```python
from build123d import *

# Parameters (mm, degrees)
SKETCH_1_W          = 35
SKETCH_1_H          = 100
EXTRUDE_1_DEPTH     = 100
SKETCH_1_3_W        = 35
SKETCH_1_3_H        = 100
EXTRUDE_2_DEPTH     = 120
SKETCH_1_4_W        = 35
SKETCH_1_4_H        = 100
EXTRUDE_3_DEPTH     = 140
SKETCH_1_5_W        = 195.279005499
SKETCH_1_5_H        = 100
EXTRUDE_4_DEPTH     = 160
SKETCH_1_6_W        = 60
SKETCH_1_6_H        = 100
EXTRUDE_5_DEPTH     = 160
SKETCH_17_R         = 3.5
CUT_EXTRUDE_4_DEPTH = 25
SKETCH_18_R         = 3.5
CUT_EXTRUDE_5_DEPTH = 25


with BuildPart() as part:
    # Sketch 1 → Extrude 1 (new body)
    with BuildSketch(Plane(origin=(0, 0, 0), x_dir=(1, 0, 0), z_dir=(0, 1, 0))):
        with Locations((17.5, 50)):
            Rectangle(SKETCH_1_W, SKETCH_1_H)
    extrude(amount=EXTRUDE_1_DEPTH)

    # Sketch 1_3 → Extrude 2 (add)
    with BuildSketch(Plane(origin=(0, 0, 0), x_dir=(1, 0, 0), z_dir=(0, 1, 0))):
        with Locations((52.5, 50)):
            Rectangle(SKETCH_1_3_W, SKETCH_1_3_H)
    extrude(amount=EXTRUDE_2_DEPTH)

    # Sketch 1_4 → Extrude 3 (add)
    with BuildSketch(Plane(origin=(0, 0, 0), x_dir=(1, 0, 0), z_dir=(0, 1, 0))):
        with Locations((87.5, 50)):
            Rectangle(SKETCH_1_4_W, SKETCH_1_4_H)
    extrude(amount=EXTRUDE_3_DEPTH)

    # Sketch 1_5 → Extrude 4 (add)
    with BuildSketch(Plane(origin=(0, 0, 0), x_dir=(1, 0, 0), z_dir=(0, 1, 0))):
        with Locations((202.639502749, 50)):
            Rectangle(SKETCH_1_5_W, SKETCH_1_5_H)
    extrude(amount=EXTRUDE_4_DEPTH)

    # Sketch 1_6 → Extrude 5 (add)
    with BuildSketch(Plane(origin=(0, 0, 0), x_dir=(1, 0, 0), z_dir=(0, 1, 0))):
        with Locations((330.279005499, 50)):
            Rectangle(SKETCH_1_6_W, SKETCH_1_6_H)
    extrude(amount=EXTRUDE_5_DEPTH)

    # Sketch 17 → Cut-Extrude 4 (cut)
    with BuildSketch(Plane(origin=(0, 120, 0), x_dir=(1, 0, 0), z_dir=(0, 1, 0))):
        with Locations(Location((53.859111314, 83.458390634, 0), (0, 0, 270))):
            Circle(SKETCH_17_R)
        with Locations(Location((53.859111314, 62.301745528, 0), (0, 0, 270))):
            Circle(SKETCH_17_R)
        with Locations(Location((53.859111314, 41.942908687, 0), (0, 0, 270))):
            Circle(SKETCH_17_R)
        with Locations(Location((53.859111314, 19.312140714, 0), (0, 0, 270))):
            Circle(SKETCH_17_R)
    extrude(amount=-CUT_EXTRUDE_4_DEPTH, mode=Mode.SUBTRACT)

    # Sketch 18 → Cut-Extrude 5 (cut)
    with BuildSketch(Plane(origin=(0, 140, 0), x_dir=(1, 0, 0), z_dir=(0, 1, 0))):
        with Locations(Location((87.572175359, 84.853566518, 0), (0, 0, 270))):
            Circle(SKETCH_18_R)
        with Locations(Location((87.572175359, 63.696921411, 0), (0, 0, 270))):
            Circle(SKETCH_18_R)
        with Locations(Location((87.572175359, 43.338084571, 0), (0, 0, 270))):
            Circle(SKETCH_18_R)
        with Locations(Location((87.572175359, 20.707316598, 0), (0, 0, 270))):
            Circle(SKETCH_18_R)
    extrude(amount=-CUT_EXTRUDE_5_DEPTH, mode=Mode.SUBTRACT)


solid = part.part
```
Design review of the part built by this model. Coordinates are the model's own, in mm. A direction names the side the tool comes from. Round coordinates to 2 decimals unless told otherwise and drop trailing zeros. Order: outer loops, then holes, each group sorted by start corner. A loop starts at its lowest first (then second) coordinate and runs counter-clockwise, first axis right, second up. Notation, with made-up numbers: M 26.25,-15.5 L 75.25,-15.5 A15 ccw 75.25,-0.5 Z; hole C 20,12.25 d5. An arc over 180 degrees is marked long. Put each result on its own line as item: value.
Q1. Draft analysis for pull direction Z (two halves, no side actions). For faces 4 (the face through (54, 95, -19)), 5 (the face through (105, 150, -49)), 6 (the face through (178, 79, -100)), state which applies: released by +Z, released by -Z, zero draft, split by the parting line, or undercut.
Reported:
face 4: undercut
face 5: zero draft
face 6: released by -Z
Q2. Consider section B-B (y = 107). State the section outline as (x, z) points.
Reported:
outline: M 35,-100 L 360.28,-100 L 360.28,0 L 35,0 Z; hole C 53.86,-83.46 d7; hole C 53.86,-62.3 d7; hole C 53.86,-41.94 d7; hole C 53.86,-19.31 d7
Q3. Consider section C-C (y = 129). State the section outline as (x, z) points.
Reported:
outline: M 70,-100 L 360.28,-100 L 360.28,0 L 70,0 Z; hole C 87.57,-84.85 d7; hole C 87.57,-63.7 d7; hole C 87.57,-43.34 d7; hole C 87.57,-20.71 d7
Q4. To check wall thickness, follow line 1 (Z direction, x = 86.5, y = 138); line 2 (Y direction, x = 87, z = -21); line 3 (X direction, y = 134, z = -67.5). State the ranges of each line that lie inside material, in increasing order.
Reported:
line 1: -100 to -88.19, -81.52 to -67.03, -60.37 to -46.67, -40.01 to -24.04, -17.38 to 0
line 2: 0 to 115
line 3: 70 to 360.28
Q5. Machinability: for faces 1 (the face through (87, 140, -51)), 2 (the face through (0, 49, -49)), 3 (the face through (89.938, 127.675, -45.918)), which of the approach directions +Z, -Z, +X, -X, +Y, -Y give a long, thin tool a straight path to every point of the face, cutting with its end or side? Answer none if there is none.
Reported:
face 1: +Z, -Z, -X, +Y
face 2: +Z, -Z, -X, +Y, -Y
face 3: +Y
Q6. Consider section A-A (z = -30). State the section outline as (x, y) points, and give its area (3 significant figures).
Reported:
outline: M 0,0 L 360.28,0 L 360.28,160 L 105,160 L 105,140 L 70,140 L 70,120 L 35,120 L 35,100 L 0,100 Z
area: 53,400 mm²
Q7. Insertion check: pin 1 Ø6 at (y, z) = (148, -49.5) entering from -X; pin 2 Ø10 at (x, z) = (66.5, -79) entering from +Y; pin 3 Ø7.5 at (x, z) = (53.5, -43) entering from +Y. Each pin has a flat end and moves straight along its axis. Give the tip position at first contact, or say it passes through.
Reported:
pin 1: x = 105
pin 2: y = 140
pin 3: y = 120
